from build123d import *

# Parameters (mm, degrees)
SKETCH1_W           = 186
SKETCH1_H           = 115.4
BOSS_EXTRUDE1_DEPTH = 10
CUT_EXTRUDE5_DEPTH  = 220.119054397
SKETCH4_W           = 166
SKETCH4_H           = 4
BOSS_EXTRUDE3_DEPTH = 6
SKETCH6_W           = 4
SKETCH6_H           = 105.4
BOSS_EXTRUDE4_DEPTH = 10
SKETCH7_W           = 4
SKETCH7_H           = 105.4
BOSS_EXTRUDE5_DEPTH = 10


with BuildPart() as part:
    # Sketch1 → Boss-Extrude1 (new body)
    with BuildSketch(Plane(origin=(0, 0, 0), x_dir=(1, 0, 0), z_dir=(0, 1, 0))):
        with Locations((93, 57.7)):
            Rectangle(SKETCH1_W, SKETCH1_H)
    extrude(amount=BOSS_EXTRUDE1_DEPTH)

    # Sketch5 → Cut-Extrude5 (cut, through all)
    with BuildSketch(Plane(origin=(0, 10, 0), x_dir=(1, 0, 0), z_dir=(0, 1, 0))):
        with BuildLine():
            Line((176, 0), (10, 0))
            ThreePointArc((10, 0), (93, 30), (176, 0))
        make_face()
    extrude(amount=-CUT_EXTRUDE5_DEPTH, mode=Mode.SUBTRACT)

    # Sketch4 → Boss-Extrude3 (add)
    with BuildSketch(Plane(origin=(0, 10, 0), x_dir=(1, 0, 0), z_dir=(0, 1, 0))):
        with Locations((93, 102.7)):
            Rectangle(SKETCH4_W, SKETCH4_H)
        with Locations((93, 110.14)):
            Rectangle(SKETCH4_W, SKETCH4_H)
    extrude(amount=BOSS_EXTRUDE3_DEPTH)

    # Sketch6 → Boss-Extrude4 (add)
    with BuildSketch(Plane(origin=(0, 10, 0), x_dir=(1, 0, 0), z_dir=(0, 1, 0))):
        with Locations((181, 57.7)):
            Rectangle(SKETCH6_W, SKETCH6_H)
    extrude(amount=BOSS_EXTRUDE4_DEPTH)

    # Sketch7 → Boss-Extrude5 (add)
    with BuildSketch(Plane(origin=(0, 10, 0), x_dir=(1, 0, 0), z_dir=(0, 1, 0))):
        with Locations((5, 57.7)):
            Rectangle(SKETCH7_W, SKETCH7_H)
    extrude(amount=BOSS_EXTRUDE5_DEPTH)


solid = part.part
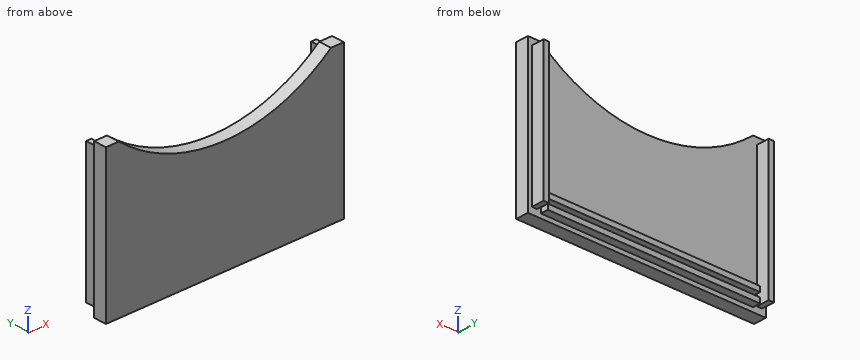
Model file for the job. Use its own axes, mm. Give positions to 0.01 mm unless a question says otherwise; leave off trailing zeros. Order: outer loops, then holes, each group sorted by start corner. A loop starts at its lowest first (then second) coordinate and runs counter-clockwise, first axis right, second up. Notation, with made-up numbers: (36.25, 49.5) - (44.25, 49.5) arc R12 cw to (44.25, 53.5) - close; hole circle Ø4 at (33.5, 75). An arc over 180 degrees is marked (long way). Write item = value, one per line. Start each with the question number.
1. Cut at D-D, the plane x = 87.5. List the corners of the cut face in (y, z), and give its area (3 significant figures).
2. Drop flat-ended pins along their axis: P1, Ø3, axis at y = 13.5, z = -110.5, coming from the +X side; P2, Ø12, axis at x = 35, z = -37.5, coming from the +Y side; P3, Ø5, axis at x = 163.5, y = 15.5, coming from the -Z side. Give the stop position or say it passes through.
3. Cut at B-B, the plane z = -53.5. List the corners of the cut face in (x, y).
4. Probe line 1 along X through (y, z) = (11.5, -13); line 2 along Z through (x, y) = (87.5, 10.25); line 3 along Y through (x, z) = (149.5, -61). List the from-to ranges inside material, lowest first.
5. Cut at C-C, the plane z = -14.5. List the corners of the cut face in (x, y), and give its area (3 significant figures).
6. Cut at A-A, the plane y = 13. List the corners of the cut face in (x, z).
Taken from the geometry:
q1.outline = (0, -115.4) - (10, -115.4) - (10, -112.14) - (16, -112.14) - (16, -108.14) - (10, -108.14) - (10, -104.7) - (16, -104.7) - (16, -100.7) - (10, -100.7) - (10, -29.88) - (0, -29.88) - close
q1.area = 903 mm²
q2.P1 = 183
q2.P2 = 10
q2.P3 = -112.14
q3.outline = (0, 0) - (186, 0) - (186, 10) - (183, 10) - (183, 20) - (179, 20) - (179, 10) - (7, 10) - (7, 20) - (3, 20) - (3, 10) - (0, 10) - close
q4.line_1 = 3 to 7, 179 to 183
q4.line_2 = -112.14 to -108.14, -104.7 to -100.7
q4.line_3 = 0 to 10
q5.outline = (0, 0) - (31.49, 0) - (31.49, 10) - (7, 10) - (7, 20) - (3, 20) - (3, 10) - (0, 10) - close; (154.51, 0) - (186, 0) - (186, 10) - (183, 10) - (183, 20) - (179, 20) - (179, 10) - (154.51, 10) - close
q5.area = 710 mm²
q6.outline = (3, -110.4) - (7, -110.4) - (7, -5) - (3, -5) - close; (10, -112.14) - (176, -112.14) - (176, -108.14) - (10, -108.14) - close; (10, -104.7) - (176, -104.7) - (176, -100.7) - (10, -100.7) - close; (179, -110.4) - (183, -110.4) - (183, -5) - (179, -5) - close
